Check sheet for the modelled part. Datum: model origin and axes. Units: mm. Face numbers are marked on the shaded views. A direction names the side the tool comes from. Give positions to 0.01 mm unless a question says otherwise; leave off trailing zeros. Write each loop counter-clockwise with the first axis right and the second up, starting at its lowest first coordinate (ties: lowest second). Pieces come first, ordered by that corner, then holes.
from build123d import *

# Parameters (mm, degrees)
SKETCH_1_W          = 60
SKETCH_1_H          = 45
EXTRUDE_1_DEPTH     = 1.5
EXTRUDE_2_DEPTH     = 96
SKETCH_4_W          = 60
SKETCH_4_H          = 2.1
EXTRUDE_3_DEPTH     = 1.5
EXTRUDE_4_DEPTH     = 1.5
CUT_EXTRUDE_2_DEPTH = 100
EXTRUDE_5_DEPTH     = 96
SKETCH_12_W         = 3
SKETCH_12_H         = 14
EXTRUDE_6_DEPTH     = 2
FILLET_1_R          = 1.5
SKETCH_13_W         = 2
SKETCH_13_H         = 5.103076436
EXTRUDE_7_DEPTH     = 1.5
FILLET_3_R          = 1
CHAMFER_3_SIZE      = 3
CHAMFER_3_SIZE2     = 1.091910703


with BuildPart() as part:
    # Эскиз1 → Бобышка-Вытянуть1 (new body)
    with BuildSketch(Plane.XY):
        Polygon((46, -35), (-46, -35), (-48, -35), (-48, -25), (-48, 25), (-48, 27), (-46, 27), (46, 27), (48, 27), (48, 25), (48, -25), (48, -35), align=None)
        Rectangle(SKETCH_1_W, SKETCH_1_H, mode=Mode.SUBTRACT)
    extrude(amount=EXTRUDE_1_DEPTH)

    # Эскиз2 → Бобышка-Вытянуть2 (add)
    with BuildSketch(Plane(origin=(48, 0, 0), x_dir=(0, 0, -1), z_dir=(1, 0, 0))):
        Polygon((8.78785553, 39.260588787), (9.668091663, 38.521982973), (0, 27), (-1.5, 27), align=None)
        Polygon((0, -32.66641426), (0, -35), (16.069690242, -15.848888922), (14.920623577, -14.884707507), align=None)
    extrude(amount=-EXTRUDE_2_DEPTH)

    # Эскиз4 → Бобышка-Вытянуть3 (add)
    with BuildSketch(Plane.XY.offset(1.5)):
        with Locations((0, 21.45)):
            Rectangle(SKETCH_4_W, SKETCH_4_H)
    extrude(amount=-EXTRUDE_3_DEPTH)

    # Эскиз6 → Бобышка-Вытянуть4 (add)
    with BuildSketch(Plane.XY.offset(1.5)):
        Polygon((-28.65, -20.7), (-28.65, 20.4), (-30, 20.4), (-30, -22.5), (-28.65, -22.5), align=None)
        Polygon((28.65, 20.4), (28.65, -20.7), (28.65, -22.5), (30, -22.5), (30, 20.4), align=None)
    extrude(amount=-EXTRUDE_4_DEPTH)

    # Эскиз8 → Вырез-Вытянуть2 (cut)
    with BuildSketch(Plane(origin=(48, 0, 0), x_dir=(0, 0, -1), z_dir=(1, 0, 0))):
        Polygon((5.785088487, 33.894399988), (4.904852354, 34.633005803), (8.78785553, 39.260588787), (9.668091663, 38.521982973), align=None)
    extrude(amount=-CUT_EXTRUDE_2_DEPTH, mode=Mode.SUBTRACT)

    # Эскиз9 → Бобышка-Вытянуть5 (add)
    with BuildSketch(Plane(origin=(48, 0, 0), x_dir=(0, 0, -1), z_dir=(1, 0, 0))):
        Polygon((-1.5, -35), (-1.5, -36.787630389), (0, -35), align=None)
    extrude(amount=-EXTRUDE_5_DEPTH)

    # Эскиз12 → Бобышка-Вытянуть6 (add)
    with BuildSketch(Plane(origin=(0, 11.155749601, 13.294904666), x_dir=(-1, 0, 0), z_dir=(0, -0.6427876096865351, -0.7660444431189816))):
        with Locations((44.5, 27.683199964)):
            Rectangle(SKETCH_12_W, SKETCH_12_H)
        with Locations((-44.5, 27.683199964)):
            Rectangle(SKETCH_12_W, SKETCH_12_H)
    extrude(amount=EXTRUDE_6_DEPTH)

    # Скругление1
    fillet_1_edges = [part.edges().sort_by_distance(p)[0] for p in [
        (-43, 31.076735882, -6.031602154),
        (-46, 31.076735882, -6.031602154),
        (-44.5, 25.714424781, -1.532088886),
        (46, 31.076735882, -6.031602154),
        (43, 31.076735882, -6.031602154),
        (44.5, 25.714424781, -1.532088886),
    ]]
    fillet(fillet_1_edges, radius=FILLET_1_R - 0.0001)  # a hair under: the kernel refuses the full size

    # Эскиз13 → Бобышка-Вытянуть7 (add)
    with BuildSketch(Plane(origin=(0, -13.496975476, -16.085069013), x_dir=(1, 0, 0), z_dir=(0, 0.642787609686538, 0.7660444431189792))):
        with Locations((-45.5, -4.363093727)):
            Rectangle(SKETCH_13_W, SKETCH_13_H)
        with Locations((45.5, -4.363093727)):
            Rectangle(SKETCH_13_W, SKETCH_13_H)
    extrude(amount=EXTRUDE_7_DEPTH)

    # Скругление3
    fillet_3_edges = [part.edges().sort_by_distance(p)[0] for p in [
        (-46.5, -15.875117766, -12.131459761),
        (-45.5, -17.82970944, -10.491362608),
        (-44.5, -15.875117766, -12.131459761),
        (-45.5, -13.920526093, -13.771556913),
        (45.5, -13.920526093, -13.771556913),
        (44.5, -15.875117766, -12.131459761),
        (45.5, -17.82970944, -10.491362608),
        (46.5, -15.875117766, -12.131459761),
    ]]
    fillet(fillet_3_edges, radius=FILLET_3_R - 0.0001)  # a hair under: the kernel refuses the full size

    # Фаска3
    chamfer_3_edges = [part.edges().sort_by_distance(p)[0] for p in [
        (28.65, -1.05, 1.5),
        (0, 20.4, 1.5),
        (0, -22.5, 1.5),
        (-28.65, -1.05, 1.5),
    ]]
    chamfer_3_side = [part.faces().sort_by_distance(p)[0] for p in [
        (-46.847400252, -4.893815194, 1.5),
    ]]
    chamfer(chamfer_3_edges, length=CHAMFER_3_SIZE, length2=CHAMFER_3_SIZE2, reference=chamfer_3_side[0])


solid = part.part
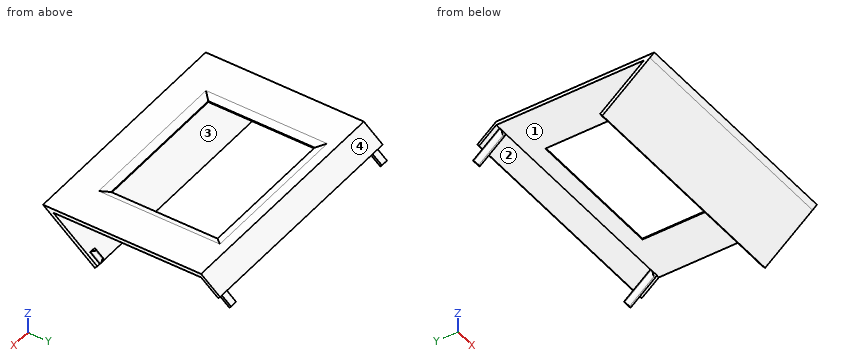
1) Draft check along X on the marked faces 1 and 2. Enter one of: +X half, -X half, draft (parallel to the pull), parting line (faces both ways), or undercut.
2) Sectioned sample at B-B on x = 6. Record the boundary of the cut face in (y, z), then the cut area to 3 significant figures.
3) Gauge pin test, flat ends, axial feed: pin 1 (8 mm diameter, centred on y = -28, z = -12.5, fed in from -X); pin 2 (10 mm diameter, centred on x = -13.5, z = -11.5, fed in from -Y); pin 3 (3 mm diameter, centred on x = 34.5, z = -9.5, fed in from +Y); pin 4 (3 mm diameter, centred on x = 29.5, z = -0.5, fed in from -Y). Record the tip position at first contact, or that the pin passes through.
4) Sectioned sample at C-C on x = 40. Record the boundary of the cut face in (y, z).
5) Access from +Z, -Z, +X, -X, +Y, -Y to the whole of each face (thin tool, end or side, straight path). Record for the marked faces 3 and 4.
6) Sectioned sample at D-D on x = 30. Record the boundary of the cut face in (y, z), then the cut area to 3 significant figures.
7) Scan lines: L1, parallel to Z at x = -17.5, y = 24.5; L2, parallel to Y at x = -2, z = -5.5; L3, parallel to Y at x = 40, z = -2.5. Record each from-to range of solid material in increasing order.
8) Sectioned sample at A-A on y = 17.5. Record the boundary of the cut face in (x, z), then the cut area to 3 significant figures.
Answers below:
1. face 1: draft
1. face 2: undercut
2. outline: (-36.79, 1.5) - (-15.85, -16.07) - (-14.88, -14.92) - (-32.67, 0) - (-22.5, 0) - (-22.5, 0.41) - (-25.5, 1.5) - close; (20.4, 0) - (27, 0) - (33.89, -5.79) - (34.63, -4.9) - (27, 1.5) - (23.4, 1.5) - (20.4, 0.41) - close
2. area: 73.8 mm2
3. pin 1: passes through
3. pin 2: stops at y = -27.25
3. pin 3: stops at y = -19.56
3. pin 4: stops at y = -36.19
4. outline: (-36.79, 1.5) - (-15.85, -16.07) - (-14.88, -14.92) - (-32.67, 0) - (27, 0) - (33.89, -5.79) - (34.63, -4.9) - (27, 1.5) - close
5. face 3: none
5. face 4: +Z, +X, -X, +Y
6. outline: (-36.79, 1.5) - (-15.85, -16.07) - (-14.88, -14.92) - (-32.67, 0) - (27, 0) - (33.89, -5.79) - (34.63, -4.9) - (27, 1.5) - (23.4, 1.5) - (21.75, 0.9) - (-23.85, 0.9) - (-25.5, 1.5) - close
6. area: 113 mm2
7. L1: z = 0 to 1.5
7. L2: y = -28.45 to -26.11, 33.55 to 34.13
7. L3: y = -32.02 to -29.69, 29.98 to 31.77
8. outline: (-48, 0) - (-28.65, 0) - (-28.65, 0.41) - (-31.65, 1.5) - (-48, 1.5) - close; (28.65, 0) - (48, 0) - (48, 1.5) - (31.65, 1.5) - (28.65, 0.41) - close
8. area: 54.8 mm2
